Verification items for the finished model (mm, model axes). Coordinates: 2 decimals unless noted, no trailing zeros. Loops run counter-clockwise (first coordinate to the right, second up) from the corner with the lowest first, then second, coordinate; pieces in that order, holes last. Notation, with made-up numbers: (88, -35) -> (103, -35) arc R22 ccw to (103, 1) -> close; hole circle Ø8 at (-2, 60). An arc over 180 degrees is marked (long way). Answer as a JSON object with one key per item and string values. Group by question number.
Q1. Scan lines: L1, parallel to X at y = -0.5, z = 2.4; L2, parallel to Y at x = 0, z = 0.6; L3, parallel to Y at x = -10.5, z = 2.4. Record each from-to range of solid material in increasing order.
Q2. Cross-section at C-C on x = 22.5. Record the boundary of the cut face in (y, z) (3 decimals), and give its area (3 significant figures).
Q3. Cross-section at A-A on x = 0. Record the boundary of the cut face in (y, z), and give its area (3 significant figures).
Q4. Release check for a two-part mould opening along X. For faces 1 (the cylindrical face through (-12.287, -10.717, 1.521)), 2 (the flat face through (14, 0, 0)), 3 (the flat face through (14.79, 15.145, 1.479)) record: released by +X, released by -X, zero draft, split by the parting line, or undercut.
Q5. Gauge pin test, flat ends, axial feed: pin 1 Ø4 at (x, y) = (10.78, 10.78) entering from -Z; pin 2 Ø1.8 at (x, y) = (-10.78, -10.78) entering from +Z; pin 3 Ø1.5 at (y, z) = (-3.5, 0.5) entering from -X. Record the tip position at first contact, or that the pin passes through.
Q6. Cross-section at B-B on y = 0. Record the boundary of the cut face in (x, z).
Q7. Cross-section at D-D on y = 10. Record the boundary of the cut face in (x, z), and give its area (3 significant figures).
```python
from build123d import *

# Parameters (mm, degrees)
SKETCH_1_R          = 12.25
EXTRUDE_1_DEPTH     = 3
SKETCH_2_R          = 1.505
CUT_EXTRUDE_1_DEPTH = 32
SKETCH_4_R          = 1.505
CUT_EXTRUDE_2_DEPTH = 3


with BuildPart() as part:
    # 草图1 → 凸台-拉伸1 (new body)
    with BuildSketch(Plane.XY):
        with BuildLine():
            Line((25.5, 12.5), (25.5, -12.5))
            Line((25.5, -12.5), (4.376204333, -17.71754316))
            ThreePointArc((4.376204333, -17.71754316), (-18.25, 0), (4.376204333, 17.71754316))
            Line((4.376204333, 17.71754316), (25.5, 12.5))
        make_face()
        Circle(SKETCH_1_R, mode=Mode.SUBTRACT)
    extrude(amount=EXTRUDE_1_DEPTH)

    # 草图2 → 切除-拉伸1 (cut)
    with BuildSketch(Plane.XY.offset(3)):
        with Locations((-10.783378413, 10.783378413)):
            Circle(SKETCH_2_R)
        with Locations((10.783378413, 10.783378413)):
            Circle(SKETCH_2_R)
        with Locations((10.783378413, -10.783378413)):
            Circle(SKETCH_2_R)
        with Locations((-10.783378413, -10.783378413)):
            Circle(SKETCH_2_R)
    extrude(amount=-CUT_EXTRUDE_1_DEPTH, mode=Mode.SUBTRACT)

    # 草图4 → 切除-拉伸2 (cut, symmetric)
    with BuildSketch(Plane.XY.offset(3)):
        with Locations((22.5, -9)):
            Circle(SKETCH_4_R)
        with Locations((22.5, 9)):
            Circle(SKETCH_4_R)
    extrude(amount=CUT_EXTRUDE_2_DEPTH, both=True, mode=Mode.SUBTRACT)


solid = part.part
```
Computed values:
{
 "1": {"L1": "x = -18.24 to -12.24, 12.24 to 25.5", "L2": "y = -18.25 to -12.25, 12.25 to 18.25", "L3": "y = -14.93 to -12.26, -9.31 to -6.31, 6.31 to 9.31, 12.26 to 14.93"},
 "2": {"outline": "(-13.241, 0) -> (-10.505, 0) -> (-10.505, 3) -> (-13.241, 3) -> close; (-7.495, 0) -> (7.495, 0) -> (7.495, 3) -> (-7.495, 3) -> close; (10.505, 0) -> (13.241, 0) -> (13.241, 3) -> (10.505, 3) -> close", "area": "61.4 mm²"},
 "3": {"outline": "(-18.25, 0) -> (-12.25, 0) -> (-12.25, 3) -> (-18.25, 3) -> close; (12.25, 0) -> (18.25, 0) -> (18.25, 3) -> (12.25, 3) -> close", "area": "36.0 mm²"},
 "4": {"face 1": "undercut", "face 2": "zero draft", "face 3": "released by +X"},
 "5": {"pin 1": "stops at z = 0", "pin 2": "passes through", "pin 3": "stops at x = -18.04"},
 "6": {"outline": "(-18.25, 0) -> (-12.25, 0) -> (-12.25, 3) -> (-18.25, 3) -> close; (12.25, 0) -> (25.5, 0) -> (25.5, 3) -> (12.25, 3) -> close"},
 "7": {"outline": "(-15.27, 0) -> (-12.07, 0) -> (-12.07, 3) -> (-15.27, 3) -> close; (-9.5, 0) -> (-7.08, 0) -> (-7.08, 3) -> (-9.5, 3) -> close; (7.08, 0) -> (9.5, 0) -> (9.5, 3) -> (7.08, 3) -> close; (12.07, 0) -> (21.38, 0) -> (21.38, 3) -> (12.07, 3) -> close; (23.62, 0) -> (25.5, 0) -> (25.5, 3) -> (23.62, 3) -> close", "area": "57.7 mm²"}
}
